Check sheet for the drawn part. Datum: minimum x, y, z corner. Units: mm. A direction names the side the tool comes from. Give positions to 0.01 mm unless a question says otherwise; leave off trailing zeros. Loops run counter-clockwise (first coordinate to the right, second up) from the corner with the lowest first, then second, coordinate; pieces in that order, holes last. Notation, with made-up numbers: (6.25, 58) -> (34.25, 58) arc R10 cw to (34.25, 62) -> close; hole circle Ø2 at (24.25, -6.5). An arc over 180 degrees is marked (long way). One line per question, with ' | ' between items.
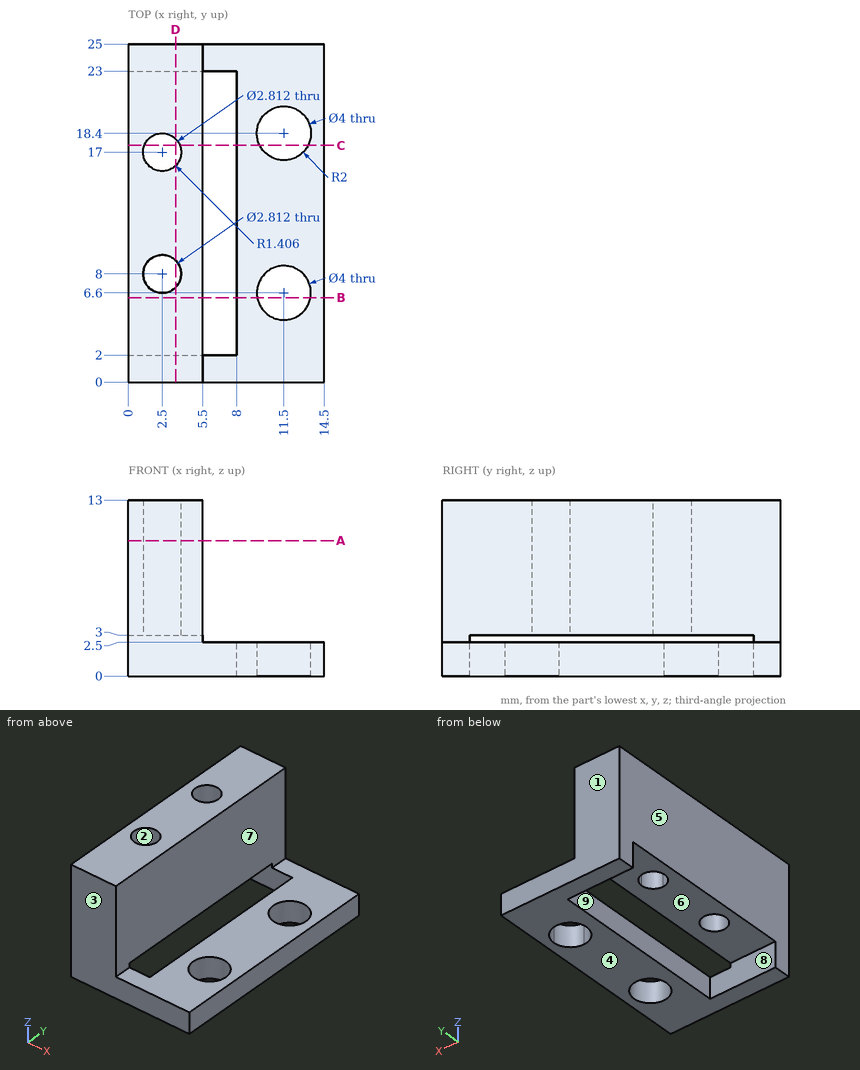
Item 1: Sectioned sample at B-B (y = 6.25). Record the cut outline in (x, z).
Result:
outline: (0, 3) -> (5.5, 3) -> (5.5, 13) -> (0, 13) -> close; (8, 0) -> (9.53, 0) -> (9.53, 2.5) -> (8, 2.5) -> close; (13.47, 0) -> (14.5, 0) -> (14.5, 2.5) -> (13.47, 2.5) -> close
Item 2: Release check for a two-part mould opening along Y. For the marked faces 1, 2, 3 and 4 record: pulls with the +Y half, pulls with the -Y half, needs draft (parallel to the pull), parting line crosses it, or undercut.
Result:
face 1: pulls with the +Y half | face 2: undercut | face 3: pulls with the -Y half | face 4: needs draft
Item 3: Sectioned sample at D-D (x = 3.5). Record the cut outline in (y, z).
Result:
outline: (0, 0) -> (2, 0) -> (2, 3) -> (7.01, 3) -> (7.01, 13) -> (0, 13) -> close; (8.99, 3) -> (16.01, 3) -> (16.01, 13) -> (8.99, 13) -> close; (17.99, 3) -> (23, 3) -> (23, 0) -> (25, 0) -> (25, 13) -> (17.99, 13) -> close
Item 4: Sectioned sample at A-A (z = 10). Record the cut outline in (x, y).
Result:
outline: (0, 0) -> (5.5, 0) -> (5.5, 25) -> (0, 25) -> close; hole circle Ø2.81 at (2.5, 8); hole circle Ø2.81 at (2.5, 17)
Item 5: Depth check by flat-ended pin: pin 1 Ø3 at (x, y) = (2.5, 16.5) entering from -Z; pin 2 Ø5 at (x, y) = (11.5, 6.6) entering from +Z; pin 3 Ø1 at (y, z) = (20.5, 9) entering from +X. Enter the tip coordinate at first touch or a pass-through.
Result:
pin 1: z = 3 | pin 2: z = 2.5 | pin 3: x = 5.5
Item 6: Sectioned sample at C-C (y = 17.5). Record the cut outline in (x, z).
Result:
outline: (0, 3) -> (1.19, 3) -> (1.19, 13) -> (0, 13) -> close; (3.81, 3) -> (5.5, 3) -> (5.5, 13) -> (3.81, 13) -> close; (8, 0) -> (9.71, 0) -> (9.71, 2.5) -> (8, 2.5) -> close; (13.29, 0) -> (14.5, 0) -> (14.5, 2.5) -> (13.29, 2.5) -> close
Item 7: Scan lines: probe 1 along Y at (x, z) = (2.5, 10.5); probe 2 along Y at (x, z) = (11.5, 1.5); probe 3 along X at (y, z) = (17, 10). Record each from-to range of solid material in increasing order.
Result:
probe 1: 0 to 6.59, 9.41 to 15.59, 18.41 to 25 | probe 2: 0 to 4.6, 8.6 to 16.4, 20.4 to 25 | probe 3: 0 to 1.09, 3.91 to 5.5
Item 8: Set-up check for the marked faces 5, 6, 7, 8 and 9: record each of +Z, -Z, +X, -X, +Y, -Y from which the full face is reachable in a straight line by a thin tool's end or side.
Result:
face 5: +Z, -Z, -X, +Y, -Y | face 6: -Z, +X, -X | face 7: +Z, +X, +Y, -Y | face 8: -Z, -X | face 9: +Z, -Z, -X
